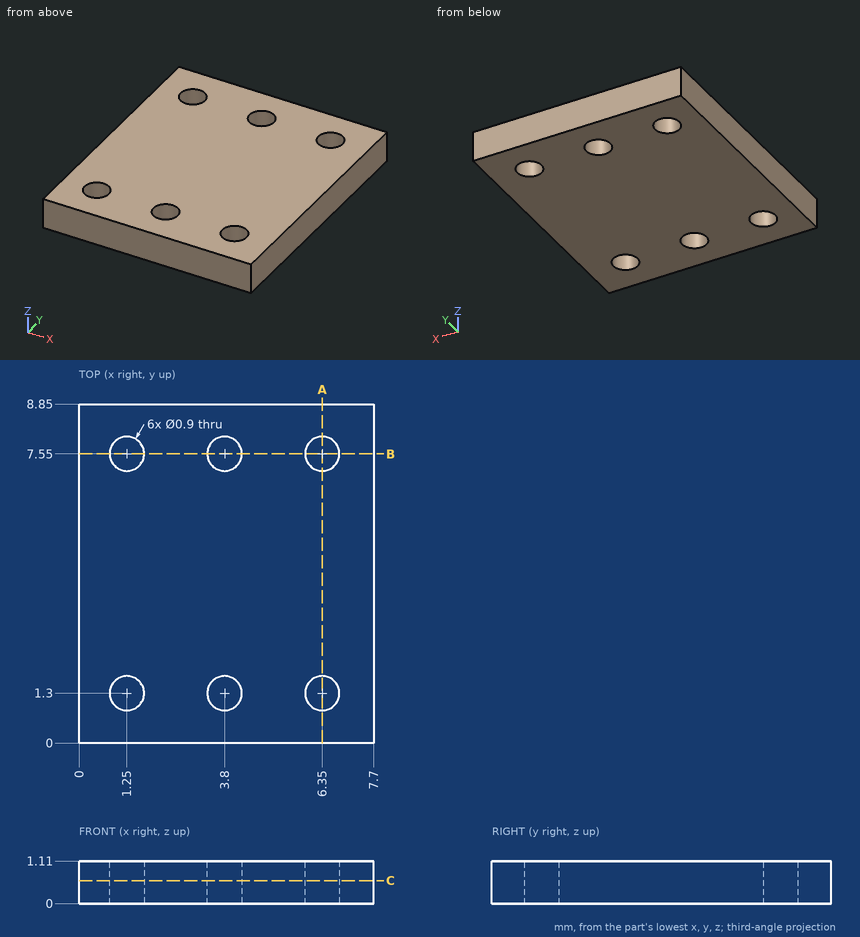
Source: three-view drawing plus pictorial views. Frame: mm from the lowest corner of the part. Give positions to 0.01 mm unless a question says otherwise; leave off trailing zeros. Order: outer loops, then holes, each group sorted by start corner. A loop starts at its lowest first (then second) coordinate and runs counter-clockwise, first axis right, second up. Notation, with made-up numbers: (30.25, 48) - (78.25, 48) arc R27 cw to (78.25, 69) - close; hole circle Ø8 at (61.5, -26.75). An arc over 180 degrees is marked (long way). Answer as a JSON object with one key per item and string values. Group by question number.
Q1. First-contact query: pin 1 Ø2 at (x, y) = (6, 5) entering from -Z. Flat tip, straight axial feed; report the tip coordinate or a pass-through.
Q2. Cut plane B-B, the plane y = 7.55. Output: boundary loops of the cut face in (x, z), then the cut area to 3 significant figures.
Q3. Line query: probe 1 along Y at (x, z) = (1.25, 0.35); probe 2 along Y at (x, z) = (3.5, 0.8). Output: solid intervals per line, ascending.
Q4. Cut plane C-C, the plane z = 0.6. Output: boundary loops of the cut face in (x, y), then the cut area to 3 significant figures.
Q5. Cut plane A-A, the plane x = 6.35. Output: boundary loops of the cut face in (y, z).
Results:
{
 "1": {"pin 1": "z = 0"},
 "2": {"outline": "(0, 0) - (0.8, 0) - (0.8, 1.11) - (0, 1.11) - close; (1.7, 0) - (3.35, 0) - (3.35, 1.11) - (1.7, 1.11) - close; (4.25, 0) - (5.9, 0) - (5.9, 1.11) - (4.25, 1.11) - close; (6.8, 0) - (7.7, 0) - (7.7, 1.11) - (6.8, 1.11) - close", "area": "5.55 mm^2"},
 "3": {"probe 1": "0 to 0.85, 1.75 to 7.1, 8 to 8.85", "probe 2": "0 to 0.96, 1.64 to 7.21, 7.89 to 8.85"},
 "4": {"outline": "(0, 0) - (7.7, 0) - (7.7, 8.85) - (0, 8.85) - close; hole circle Ø0.9 at (1.25, 1.3); hole circle Ø0.9 at (1.25, 7.55); hole circle Ø0.9 at (3.8, 1.3); hole circle Ø0.9 at (3.8, 7.55); hole circle Ø0.9 at (6.35, 1.3); hole circle Ø0.9 at (6.35, 7.55)", "area": "64.3 mm^2"},
 "5": {"outline": "(0, 0) - (0.85, 0) - (0.85, 1.11) - (0, 1.11) - close; (1.75, 0) - (7.1, 0) - (7.1, 1.11) - (1.75, 1.11) - close; (8, 0) - (8.85, 0) - (8.85, 1.11) - (8, 1.11) - close"}
}
